from build123d import *

# Parameters (mm, degrees)
F1_START = 2
F1_DEPTH = 3
F3_DEPTH = 0.4


# Not quite as in the source:
# - a pattern or mirror of a feature is missing from the dataset's text; its kind, count and spacing are read off the source's solid


with BuildPart() as f1:
    # F0 (on Top) → F1 (new body)
    with BuildSketch(Plane.XY.offset(F1_START)):
        with BuildLine():
            Line((10, 3.61), (-10, 3.61))
            Line((-10, 3.61), (-10, 1))
            ThreePointArc((-10, 1), (-9, 0), (-10, -1))
            Line((-10, -1), (-10, -3.61))
            Line((-10, -3.61), (10, -3.61))
            Line((10, -3.61), (10, 3.61))
        make_face()
    extrude(amount=F1_DEPTH)

    # F2 (on face) → F3 (join)
    with BuildSketch(Plane.XZ.offset(3.61)):
        Polygon((-6.87, 3.7), (-8.37, 3.7), (-8.37, 0.5), (-7.87, 0), (-7.87, -3), (-7.37, -3), (-7.37, 0), (-6.87, 0.5), align=None)
        Polygon((-5.83, 0.5), (-5.33, 0), (-5.33, -3), (-4.83, -3), (-4.83, 0), (-4.33, 0.5), (-4.33, 3.7), (-5.83, 3.7), align=None)
        Polygon((-3.29, 0.5), (-2.79, 0), (-2.79, -3), (-2.29, -3), (-2.29, 0), (-1.79, 0.5), (-1.79, 3.7), (-3.29, 3.7), align=None)
        Polygon((-0.75, 0.5), (-0.25, 0), (-0.25, -3), (0.25, -3), (0.25, 0), (0.75, 0.5), (0.75, 3.7), (-0.75, 3.7), align=None)
        Polygon((1.79, 0.5), (2.29, 0), (2.29, -3), (2.79, -3), (2.79, 0), (3.29, 0.5), (3.29, 3.7), (1.79, 3.7), align=None)
        Polygon((4.33, 0.5), (4.83, 0), (4.83, -3), (5.33, -3), (5.33, 0), (5.83, 0.5), (5.83, 3.7), (4.33, 3.7), align=None)
        Polygon((6.87, 0.5), (7.37, 0), (7.37, -3), (7.87, -3), (7.87, 0), (8.37, 0.5), (8.37, 3.7), (6.87, 3.7), align=None)
    f3 = extrude(amount=F3_DEPTH)

    # F3_copies: F3 across plane
    add(f3.mirror(Plane.ZX))


solid = f1.part
The listing builds one solid part. Answer for the finished solid, in the listing's coordinates (mm). A direction names the side the tool comes from. Round coordinates to 2 decimals unless told otherwise and drop trailing zeros. Loops run counter-clockwise (first coordinate to the right, second up) from the corner with the lowest first, then second, coordinate; pieces in that order, holes last. Notation, with made-up numbers: M 32,-10.5 L 83,-10.5 A20 cw 83,17.5 Z; hole C 63,57.5 d9. An arc over 180 degrees is marked long. Write each question's results on one line, items separated by ' | '. Start each with the question number.
1) Find section D-D on y = 0. Write down the section's boundary in (x, z), plus the area to 3 significant figures.
2) Find section A-A on z = 0.75. Count the separate pieces of the cut face and the enclosed holes in it, plus the area to 3 significant figures.
3) Find section B-B on y = -2. Write down the section's boundary in (x, z).
4) Straight lines are drawn through the part: probe 1 along Y at (x, z) = (7.5, -0.5); probe 2 along Z at (x, y) = (7.75, -3.5); probe 3 along Y at (x, z) = (3.75, 4.5). For each, find the intervals that lie inside material, in ascending order.
5) Determine the mould class of faces 1 (the flat face through (0, 3.61, 4)), 2 (the cylindrical face through (-9, 0, 3)), 3 (the flat face through (-3, 4.01, 1)) for opening direction X: pulls with the +X half, pulls with the -X half, needs draft (parallel to the pull), parting line crosses it, or undercut.
6) Which of the six approach directions +Z, -Z, +X, -X, +Y, -Y give full straight-line access (tool end or side, diameter ignored) to faces 4 (the flat face through (-5, -4.01, 1)), 5 (the flat face through (0, -3.61, 0))?
Final values:
1) outline: M -9,2 L 10,2 L 10,5 L -9,5 Z | area: 57.0 mm²
2) separate pieces: 14 | enclosed holes: 0 | area: 8.40 mm²
3) outline: M -10,2 L 10,2 L 10,5 L -10,5 Z
4) probe 1: -4.01 to -3.61, 3.61 to 4.01 | probe 2: 2 to 5 | probe 3: -3.61 to 3.61
5) face 1: undercut | face 2: pulls with the -X half | face 3: needs draft
6) face 4: +Z, -Z, +X, -X, -Y | face 5: -Z, +X, -X
